Here's how the part is built. I have some questions about the finished solid (model axes, mm). Face numbers are marked on the shaded views. A direction names the side the tool comes from. Round coordinates to 2 decimals unless told otherwise and drop trailing zeros. Write each loop counter-clockwise with the first axis right and the second up, starting at its lowest first coordinate (ties: lowest second). Pieces come first, ordered by that corner, then holes. Notation, with made-up numbers: (66.25, -37.75) -> (83.25, -37.75) arc R11 cw to (83.25, -16.75) -> close; hole circle Ø2 at (-28.75, 45). An arc over 180 degrees is marked (long way). Put each result on its own line as item: value. Start each with the question number.
1) I want a section at D-D, the plane z = -14.5. List the corners of the cut face in (x, y) for me.
2) Which directions (+Z, -Z, +X, -X, +Y, -Y) give clear straight access to the entire face, cutting with the end or side of a thin tool? Please do the marked faces 1 and 2.
3) I want a section at A-A, the plane z = 43.5. List the corners of the cut face in (x, y) for me.
4) If I drill on line 1 along Y through (x, z) = (29.5, -30.5); line 2 along Z through (x, y) = (33.5, 4); line 3 along Y through (x, z) = (9.5, -19), over which ranges is the centre line in solid material (lowest first)? Write a range as [from, to].
5) I want a section at B-B, the plane y = 33. List the corners of the cut face in (x, z) for me.
6) I want a section at C-C, the plane z = 10. List the corners of the cut face in (x, y) for me, then the cut area to 3 significant figures.
7) Will these pins go through, and if not, where does the flat tip stop? P1, Ø1.5, axis at y = 28.5, z = 14.5, coming from the -X side; P2, Ø21.5, axis at x = 20.5, z = -24, coming from the +Y side; P3, Ø1.6, axis at y = -1, z = 44, coming from the -X side; P4, Ø14.5, axis at y = 23, z = 29.5, coming from the -X side.
from build123d import *

# Parameters (mm, degrees)
BOSS_EXTRUDE1_DEPTH = 50
SKETCH3_W           = 3.3
SKETCH3_H           = 1
BOSS_EXTRUDE2_DEPTH = 13
BOSS_EXTRUDE3_DEPTH = 57
SKETCH6_W           = 2
SKETCH6_H           = 30
BOSS_EXTRUDE4_DEPTH = 2
CHAMFER1_START      = -14
CHAMFER1_OUTLINE_W  = 52
CHAMFER1_OUTLINE_H  = 13
CHAMFER1_DEPTH      = 3.182909169
CHAMFER2_SIZE       = 3


with BuildPart() as part:
    # Sketch2 → Boss-Extrude1 (new body)
    with BuildSketch(Plane(origin=(0, 0, 0), x_dir=(1, 0, 0), z_dir=(0, 1, 0))):
        Polygon((-1.7, -2), (-1.7, -15), (-5.7, -15), (-5.7, -2), (-9, -2), (-9, -15), (-13, -15), (-13, 2.680601608), align=None)
    extrude(amount=BOSS_EXTRUDE1_DEPTH)

    # Sketch3 → Boss-Extrude2 (add)
    with BuildSketch(Plane.XY.offset(2)):
        with Locations((-7.35, 0.5)):
            Rectangle(SKETCH3_W, SKETCH3_H)
    extrude(amount=BOSS_EXTRUDE2_DEPTH)

    # Sketch5 → Boss-Extrude3 (add)
    with BuildSketch(Plane.XY.offset(15)):
        Polygon((-13, 0), (-1.7, 0), (-1.7, 14), (-5.7, 14), (-5.7, 1), (-9, 1), (-9, 14), (-13, 14), align=None)
    extrude(amount=BOSS_EXTRUDE3_DEPTH)

    # Sketch6 → Boss-Extrude4 (add)
    with BuildSketch(Plane(origin=(0, 0, 0), x_dir=(-1, 0, 0), z_dir=(0, -1, 0))):
        with Locations((5.2, -40)):
            Rectangle(SKETCH6_W, SKETCH6_H)
        with Locations((9.5, -40)):
            Rectangle(SKETCH6_W, SKETCH6_H)
    extrude(amount=BOSS_EXTRUDE4_DEPTH)

    # Mirror1: part across plane


with BuildPart() as part_1:
    add(part.part)
    add(part.part.mirror(Plane(origin=(-0.956063716, 0, 2.308147732), x_dir=(0.9238798691632129, 0, 0.38268261961443256), z_dir=(0.3826826196144326, 0, -0.9238798691632131))))

    # Chamfer1: read off the stored shape, not the designer's step
    # Chamfer1 outline → Chamfer1 (cut)
    with BuildSketch(Plane(origin=(0, 0, 0), x_dir=(0, 1, 0), z_dir=(0.9238798691632129, 0, 0.38268261961443295)).offset(CHAMFER1_START)):
        with Locations((25, 2.5)):
            Rectangle(CHAMFER1_OUTLINE_W, CHAMFER1_OUTLINE_H)
    extrude(amount=CHAMFER1_DEPTH, mode=Mode.SUBTRACT)

    # Chamfer2
    chamfer2_edges = [part_1.edges().sort_by_distance(p)[0] for p in [
        (-13, 32, 15),
        (-13, 14, 43.5),
        (-0.497948704, 32, -15.182696898),
        (19.654559103, 14, -35.335275619),
    ]]
    chamfer(chamfer2_edges, length=CHAMFER2_SIZE)


solid = part_1.part
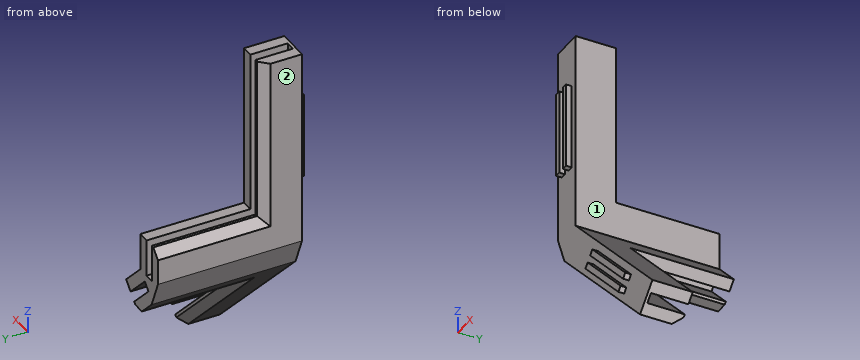
Findings:
1. outline: (-1.18, 0) -> (14.8, 0) -> (14.8, 14) -> (9.14, 14) -> (9.14, 1) -> (4.48, 1) -> (4.48, 14) -> (3.06, 14) -> (-1.18, 11) -> close
2. face 1: +Z, +X, +Y, -Y
2. face 2: +Z, -Z, -X, +Y, -Y
3. outline: (-13, 0) -> (-10.5, 0) -> (-10.5, -2) -> (-8.5, -2) -> (-8.5, 0) -> (-6.2, 0) -> (-6.2, -2) -> (-4.2, -2) -> (-4.2, 0) -> (-1.7, 0) -> (-1.7, 14) -> (-5.7, 14) -> (-5.7, 1) -> (-9, 1) -> (-9, 14) -> (-10, 14) -> (-13, 11) -> close
4. line 1: y = [0, 14]
4. line 2: z = [-49.18, -43.52], [-38.86, -33.2]
4. line 3: y = [0, 1]
5. outline: (-13, 3.12) -> (-8.9, -6.78) -> (-2.62, -13.06) -> (1.62, -13.06) -> (2.33, -12.35) -> (-6.86, -3.16) -> (-4.53, -0.83) -> (4.66, -10.02) -> (7.49, -7.19) -> (-1.7, 2) -> (-1.7, 15) -> (-5.7, 15) -> (-5.7, 2) -> (-9, 2) -> (-9, 15) -> (-10, 15) -> (-13, 12) -> close
6. outline: (-13, 0) -> (-1.7, 0) -> (-1.7, 50) -> (-5.7, 50) -> (-5.7, 1) -> (-9, 1) -> (-9, 50) -> (-13, 50) -> close
6. area: 403 mm2
7. P1: stops at x = -11.25
7. P2: stops at y = 14
7. P3: stops at x = -10.5
7. P4: passes through
